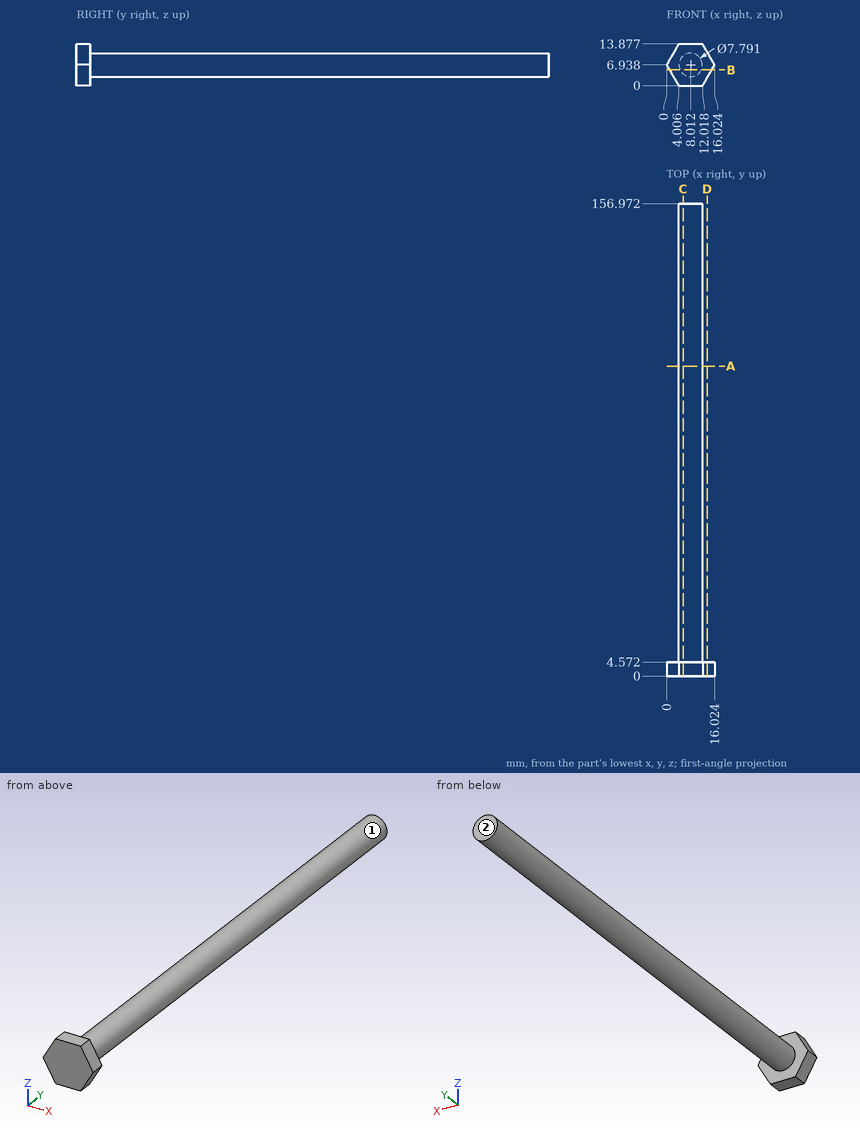
Job drawing, mm, ordinate dimensions from the low corner. One solid piece. A direction names the side the tool comes from. Coordinates: 2 decimals unless noted, no trailing zeros. Order: outer loops, then holes, each group sorted by start corner. A loop starts at its lowest first (then second) coordinate and runs counter-clockwise, first axis right, second up. Notation, with made-up numbers: (68, 51.25) - (85, 51.25) arc R24 ccw to (85, 84.25) - close; hole circle Ø8 at (-23, 59). An arc over 180 degrees is marked (long way). Use CSV: the item, a comma, the result in double quotes.
Item 1: 3-axis set-ups, long thin cutter, end or side, ignore diameter. For the marked faces 1 and 2: which of +Z, -Z, +X, -X, +Y, -Y reach the whole face in a straight line?
Solved:
face 1,"+Y"
face 2,"+Z, -Z, +X, -X, +Y"
Item 2: Saw through at A-A on y = 103. Give the cut face in (x, z) (1 decimal).
Solved:
outline,"circle Ø7.8 at (8, 6.9)"
Item 3: Drop flat-ended pins along their axis: P1, Ø1, axis at x = 8.5, y = 25.5, coming from the +Z side; P2, Ø8, axis at y = 39.5, z = 2, coming from the -X side; P3, Ø8, axis at x = 14, y = 130.5, coming from the -Z side. Give the stop position or say it passes through.
Solved:
P1,"stops at z = 10.83"
P2,"stops at x = 4.23"
P3,"stops at z = 3.59"
Item 4: Saw through at C-C on x = 5.5. Give the cut face in (y, z) (1 decimal).
Solved:
outline,"(0, 0) - (4.6, 0) - (4.6, 4) - (157, 4) - (157, 9.9) - (4.6, 9.9) - (4.6, 13.9) - (0, 13.9) - close"
Item 5: Saw through at D-D on x = 13.5. Give the cut face in (y, z).
Solved:
outline,"(0, 2.57) - (4.57, 2.57) - (4.57, 11.31) - (0, 11.31) - close"
Item 6: Probe probe 1 along Y at (x, z) = (5, 0.75); probe 2 along Z at (x, y) = (8.5, 23); probe 3 along X at (y, z) = (29.5, 9.5) (1 decimal). List the from-to ranges inside material, lowest first.
Solved:
probe 1,"y = 0 to 4.57"
probe 2,"z = 3.07 to 10.8"
probe 3,"x = 5.1 to 10.9"
Item 7: Saw through at B-B on z = 5.25. Give the cut face in (x, y) (1 decimal).
Solved:
outline,"(1, 0) - (15, 0) - (15, 4.6) - (11.5, 4.6) - (11.5, 157) - (4.5, 157) - (4.5, 4.6) - (1, 4.6) - close"
